The model under review builds one solid part; all positions refer to its coordinate system, in mm. A direction names the side the tool comes from. Coordinates: 2 decimals unless noted, no trailing zeros. Order: outer loops, then holes, each group sorted by start corner. A loop starts at its lowest first (then second) coordinate and runs counter-clockwise, first axis right, second up. Notation, with made-up numbers: (42.5, 58) -> (60.5, 58) arc R31 ccw to (60.5, 83) -> close; hole circle Ø9 at (22.25, 64.25). An arc over 180 degrees is marked (long way). Use one line per item in the form item = value.
from build123d import *

# Parameters (mm, degrees)
BF_BODY_DEPTH                = 10
BALL_BEARING_HOLE_DEPTH      = 39.522720569
BALL_BEARING_HOLE_DEPTH_BACK = 39.522720569
BALL_BEARING_HOLE_SKETCH_R   = 11
VERTICAL_HOLES_AT_2_COUNT    = 2
VERTICAL_HOLES_AT_2_PITCH    = 46
HORIZONTAL_HOLES_AT_2_COUNT  = 2
HORIZONTAL_HOLES_AT_2_PITCH  = 46
HORIZONTAL_HOLES_AT_3_COUNT  = 2
HORIZONTAL_HOLES_AT_3_PITCH  = 48.383881614
HORIZONTAL_HOLES_AT_4_COUNT  = 2
HORIZONTAL_HOLES_AT_4_PITCH  = 15
PRODUCTION_FILET_R           = 0.1
AESTHETIC_CHAMFER_SIZE       = 0.5


with BuildPart() as part:
    # BF Body Sketch → BF Body (new, symmetric)
    with BuildSketch(Plane.XY):
        Polygon((30, -22), (-30, -22), (-30, 10.5), (-17, 10.5), (-17, 17), (17, 17), (17, 10.5), (30, 10.5), align=None)
    extrude(amount=BF_BODY_DEPTH, both=True)

    # Ball Bearing Hole Sketch → Ball Bearing Hole (cut, two sides: drawn at the far end of the back side and taken through both)
    with BuildSketch(Plane.XY.offset(-BALL_BEARING_HOLE_DEPTH_BACK)):
        Circle(BALL_BEARING_HOLE_SKETCH_R)
    extrude(amount=BALL_BEARING_HOLE_DEPTH + BALL_BEARING_HOLE_DEPTH_BACK, mode=Mode.SUBTRACT)

    # Sketch2 → Vertical Holes (revolve, cut)
    with BuildSketch(Plane(origin=(-23, 10.5, 0), x_dir=(0, 0, 1), z_dir=(1, 0, 0))):
        Polygon((0, 0), (0, 32.5), (3.8, 32.5), (3.3, 32), (3.3, 5.25), (3.55, 5), (5.4, 5), (5.4, 0.5), (5.9, 0), align=None)
    vertical_holes = revolve(axis=Axis((-23, 16.85, 0), (0, -1, 0)), mode=Mode.SUBTRACT)

    # Vertical Holes at 2: Vertical Holes ×2
    with Locations(*[(i * VERTICAL_HOLES_AT_2_PITCH, 0, 0) for i in range(1, VERTICAL_HOLES_AT_2_COUNT)]):
        add(vertical_holes, mode=Mode.SUBTRACT)

    # Sketch4 → Horizontal Holes (revolve, cut)
    with BuildSketch(Plane(origin=(-23, 0, 10), x_dir=(0, -1, 0), z_dir=(1, 0, 0))):
        Polygon((0, 0), (0, 20), (3.25, 20), (2.75, 19.5), (2.75, 0.5), (3.25, 0), align=None)
    horizontal_holes = revolve(axis=Axis((-23, 0, 16.35), (0, 0, -1)), mode=Mode.SUBTRACT)

    # Horizontal Holes at 2: Horizontal Holes ×2
    with Locations(*[(i * HORIZONTAL_HOLES_AT_2_PITCH, 0, 0) for i in range(1, HORIZONTAL_HOLES_AT_2_COUNT)]):
        add(horizontal_holes, mode=Mode.SUBTRACT)

    # Horizontal Holes at 3: Horizontal Holes ×2
    with Locations(*[Vector(0.9507298394814789, -0.31002059983091673, 0) * (i * HORIZONTAL_HOLES_AT_3_PITCH) for i in range(1, HORIZONTAL_HOLES_AT_3_COUNT)]):
        add(horizontal_holes, mode=Mode.SUBTRACT)

    # Horizontal Holes at 4: Horizontal Holes ×2
    with Locations(*[(0, -i * HORIZONTAL_HOLES_AT_4_PITCH, 0) for i in range(1, HORIZONTAL_HOLES_AT_4_COUNT)]):
        add(horizontal_holes, mode=Mode.SUBTRACT)

    # Production Filet
    production_filet_edges = [part.edges().sort_by_distance(p)[0] for p in [
        (-17, 10.5, 0),
        (17, 10.5, 0),
        (23, 5.5, -5.4),
        (-23, 5.5, -5.4),
    ]]
    fillet(production_filet_edges, radius=PRODUCTION_FILET_R - 0.0001)  # a hair under: the kernel refuses the full size

    # Aesthetic Chamfer
    aesthetic_chamfer_edges = [part.edges().sort_by_distance(p)[0] for p in [
        (-23.54995, 10.5, -10),
        (-23.54995, 10.5, 10),
        (23.54995, 10.5, -10),
        (17, 13.79995, -10),
        (17, 13.79995, 10),
        (30, -5.75, -10),
        (-17.029260033, 10.529260033, -10),
        (-17.029260033, 10.529260033, 10),
        (17.029260033, 10.529260033, -10),
        (17.029260033, 10.529260033, 10),
        (0, 17, 10),
        (30, -22, 0),
        (-30, -22, 0),
        (-30, 10.5, 0),
        (-17, 17, 0),
        (17, 17, 0),
        (30, 10.5, 0),
        (-17, 13.79995, 10),
        (-30, -5.75, 10),
        (-11, 0, -10),
        (-11, 0, 10),
        (0, -22, 10),
        (30, -5.75, 10),
        (23.54995, 10.5, 10),
        (0, -22, -10),
        (-30, -5.75, -10),
        (-17, 13.79995, -10),
        (0, 17, -10),
    ]]
    chamfer(aesthetic_chamfer_edges, length=AESTHETIC_CHAMFER_SIZE)


solid = part.part
Item 1: Draft analysis for pull direction X (two halves, no side actions). For faces 4 (the face through (29, 10.5, 2)), 5 (the face through (18.447, 7.831, 2.903)), 6 (the face through (-17, 14, 0)), 7 (the face through (-23.121, 2.747, -6.461)), state which applies: released by +X, released by -X, zero draft, split by the parting line, or undercut.
Results found:
face_4 = zero draft
face_5 = undercut
face_6 = released by -X
face_7 = undercut
Item 2: We need section A-A (y = -15). State how many separate pieces and enclosed holes the cut face has, plus the area to 3 significant figures.
Results found:
separate_pieces = 3
enclosed_holes = 0
area = 973 mm²
Item 3: Clearance check with flat-ended pins moving along their axes: pin 1 (10 mm diameter, centred on x = -24.5, z = -2, fed in from +Y); pin 2 (1.8 mm diameter, centred on y = 12.5, z = 2, fed in from +X). State where each tip first meets the part, or that it passes through.
Results found:
pin_1 = 10.5
pin_2 = 17
Item 4: To check wall thickness, follow L1, parallel to X at y = -15, z = -6.25; L2, parallel to Y at x = -23, z = 4.25; L3, parallel to Y at x = -23, z = -7.75. State the ranges of each line that lie inside material, in increasing order. Write a range as from..to.
Results found:
L1 = -30..-25.75, -20.25..20.25, 25.75..30
L2 = -22..-17.75, -12.25..-2.75, 2.75..5.5
L3 = -22..-17.75, -12.25..-2.75, 2.75..10.5
Item 5: We need section C-C (z = -7.75). Write out the cut boundary in (x, y).
Results found:
outline = (-30, -21.5) -> (-29.5, -22) -> (29.5, -22) -> (30, -21.5) -> (30, 10) -> (29.5, 10.5) -> (17.1, 10.5) arc R0.1 cw to (17, 10.6) -> (17, 16.5) -> (16.5, 17) -> (-16.5, 17) -> (-17, 16.5) -> (-17, 10.6) arc R0.1 cw to (-17.1, 10.5) -> (-29.5, 10.5) -> (-30, 10) -> close; hole circle Ø5.5 at (-23, -15); hole circle Ø5.5 at (-23, 0); hole circle Ø22 at (0, 0); hole circle Ø5.5 at (23, -15); hole circle Ø5.5 at (23, 0)
Item 6: Tool access review of faces 1 (the face through (26.5, 5.5, 1.3)), 2 (the face through (20.217, -7.938, 1.774)), 3 (the face through (-29, 10.5, -2)): name each direction out of +Z, -Z, +X, -X, +Y, -Y from which nothing blocks a thin tool from reaching the whole face with its end or side.
Results found:
face_1 = +Y
face_2 = +Y, -Y
face_3 = +Z, -Z, -X, +Y
Item 7: We need section B-B (x = 0). Write out the cut boundary in (y, z).
Results found:
outline = (-22, -9.5) -> (-21.5, -10) -> (-11.5, -10) -> (-11, -9.5) -> (-11, 9.5) -> (-11.5, 10) -> (-21.5, 10) -> (-22, 9.5) -> close; (11, -9.5) -> (11.5, -10) -> (16.5, -10) -> (17, -9.5) -> (17, 9.5) -> (16.5, 10) -> (11.5, 10) -> (11, 9.5) -> close
